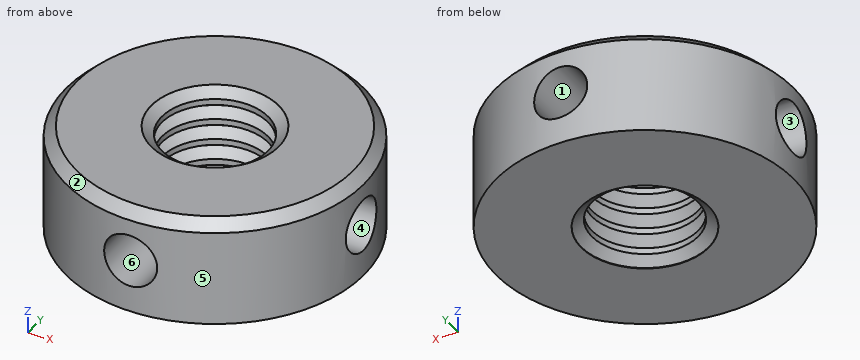
from build123d import *

# Parameters (mm, degrees)
BASENUTSKE_R    = 7
BASENUTSKE_R_2  = 2.5
BASENUT_DEPTH   = 5
HOLES_COUNT     = 4
THDSCHPAT_COUNT = 6
THDSCHPAT_PITCH = 0.98984


with BuildPart() as part:
    # BaseNutSke → BaseNut (new body)
    with BuildSketch(Plane.XY):
        Circle(BASENUTSKE_R)
        Circle(BASENUTSKE_R_2, mode=Mode.SUBTRACT)
    extrude(amount=-BASENUT_DEPTH)

    # Chamfer1: read off the stored shape, not the designer's step
    # Chamfer1 outline → Chamfer1 (revolve, cut)
    with BuildSketch(Plane.XZ):
        Polygon((2.5, 0), (2.5, -0.350103769), (3, 0), align=None)
        Polygon((7, 0), (6.5, 0), (7, -0.5), align=None)
        Polygon((3, -4.9746), (2.5, -4.624496231), (2.5, -5), (3, -5), align=None)
    revolve(axis=Axis((0, 0, 0), (0, 0, 1)), mode=Mode.SUBTRACT)

    # HoleSke → Hole (revolve, cut)
    with BuildSketch(Plane(origin=(0, 0, 0), x_dir=(0, 0, -1), z_dir=(1, 0, 0)), mode=Mode.PRIVATE) as hole_sk:
        Polygon((2.5, 7), (2.5, 3.282233047), (3.75, 3.8), (3.75, 7), align=None)
    hole = revolve(hole_sk.sketch.rotate(Axis((0, 4.7625, -2.5), (0, -1, 0)), 180), axis=Axis((0, 4.7625, -2.5), (0, -1, 0)), mode=Mode.SUBTRACT)

    # Holes: Hole ×4 about axis
    holes_axis = Axis((0, 0, 0), (0, 0, 1))
    for i in range(1, HOLES_COUNT):
        add(hole.rotate(holes_axis, i * 360 / HOLES_COUNT), mode=Mode.SUBTRACT)

    # ThdSchSke → ThreadSchematic (revolve, cut)
    with BuildSketch(Plane(origin=(0, 0, 0), x_dir=(1, 0, 0), z_dir=(0, 1, 0)), mode=Mode.PRIVATE) as threadschematic_sk:
        Polygon((-3, 0.025), (-2.5, 0.375103769), (-1.25, 0.375103769), (-1.25, -0.325103769), (-2.5, -0.325103769), align=None)
    threadschematic = revolve(threadschematic_sk.sketch.rotate(Axis((0, 0, -0.525), (0, 0, -1)), 180), axis=Axis((0, 0, -0.525), (0, 0, -1)), mode=Mode.SUBTRACT)

    # ThdSchPat: ThreadSchematic ×6
    with Locations(*[(0, 0, -i * THDSCHPAT_PITCH) for i in range(1, THDSCHPAT_COUNT)]):
        add(threadschematic, mode=Mode.SUBTRACT)


solid = part.part
Here's how the part is built. I have some questions about the finished solid (model axes, mm). Face numbers are marked on the shaded views. A direction names the side the tool comes from. Round coordinates to 2 decimals unless told otherwise and drop trailing zeros. Order: outer loops, then holes, each group sorted by start corner. A loop starts at its lowest first (then second) coordinate and runs counter-clockwise, first axis right, second up. Notation, with made-up numbers: M 15.5,88.25 L 30.5,88.25 A20 cw 30.5,126.25 Z; hole C -26,-32.5 d9. An arc over 180 degrees is marked long. One line per question, with ' | ' between items.
1) Imagine slicing it at A-A, the plane z = -0.85. Write out the boundary of the cut face in (x, y).
Checked values:
outline: C 0,0 d14; hole C 0,0 d5.53
2) On a 3-axis mill with a long thin cutter (end or side, diameter ignored), from which of +Z, -Z, +X, -X, +Y, -Y can I reach the whole of each face in a straight line? I mean the marked faces 4, 5 and 6. Say none if no direction works.
Checked values:
face 4: +X | face 5: +Z, -Z | face 6: -Y
3) We'd pull the mould along Y, two halves only. Please class the marked faces 1, 2 and 3: released by +Y, released by -Y, zero draft, split by the parting line, or undercut.
Checked values:
face 1: zero draft | face 2: split by the parting line | face 3: undercut
4) I need wall thicknesses on line 1 (Y direction, x = 0, z = -4.5); line 2 (Z direction, x = 0, y = 2.75); line 3 (X direction, y = -5, z = -2.45). Which ranges of each line are inside material? Lowest first, please.
Checked values:
line 1: y = -7 to -2.5, 2.5 to 7 | line 2: z = -4.8 to -4.16, -3.81 to -3.17, -2.82 to -2.18, -1.83 to -1.19, -0.84 to -0.2 | line 3: x = -4.9 to -1.25, 1.25 to 4.9
5) I'm going to push flat-ended pins straight in: pin 1 Ø3 at (y, z) = (-4, -3) entering from -X; pin 2 Ø2 at (x, z) = (-2, -1.5) entering from +Y; pin 3 Ø1.5 at (y, z) = (0, -2.5) entering from +X. Where does each tip first touch, or does it pass through?
Checked values:
pin 1: stops at x = -6.54 | pin 2: stops at y = 6.93 | pin 3: stops at x = 3.59
